Here's how the part is built. I have some questions about the finished solid (model axes, mm). A direction names the side the tool comes from. Round coordinates to 2 decimals unless told otherwise and drop trailing zeros. Write each loop counter-clockwise with the first axis right and the second up, starting at its lowest first coordinate (ties: lowest second). Pieces come first, ordered by that corner, then holes. Notation, with made-up numbers: (-37.75, -8.75) -> (17.25, -8.75) arc R14 ccw to (17.25, 7.25) -> close; hole circle Ø1 at (48, 10). An arc over 180 degrees is marked (long way). Put each result on its own line as item: value. Start each with the question number.
1. Suppose I cut it at D-D (x = 0). Please give me the cut outline in (y, z), then the cut area to 3 significant figures.
2. I need wall thicknesses on probe 1 along Y at (x, z) = (-7.25, -5.25); probe 2 along Y at (x, z) = (4.5, 4.5); probe 3 along X at (y, z) = (29, 0.25). Which ranges of each line are inside material? Lowest first, please. Write a range as from..to.
3. Suppose I cut it at B-B (z = 0). Please give me the cut outline in (x, y), then the cut area to 3 significant figures.
4. Which directions (+Z, -Z, +X, -X, +Y, -Y) give clear straight access to the entire face, cutting with the end or side of a thin tool? Please do faces 1 (the face through (0, 0, 0)), 2 (the face through (-6.324, 8.381, -4.032)), 3 (the face through (3, 47.5, 3)).
5. For pin 1 (4 mm diameter, centred on y = 62.5, z = 0, fed in from +X); pin 2 (4 mm diameter, centred on x = 6, y = 23.5, fed in from +Z); pin 3 (2 mm diameter, centred on y = 48, z = 2.5, fed in from +X), each with a flat end and sliding along its axis, tell me the tip position at first contact or that it passes through.
6. Suppose I cut it at C-C (y = 44.5). Please give me the cut outline in (x, z), then the cut area to 3 significant figures.
7. Suppose I cut it at A-A (x = -6). Please give me the cut outline in (y, z), then the cut area to 3 significant figures.
```python
from build123d import *


with BuildPart() as part:
    # Szkic1 → Obrót1 (revolve)
    with BuildSketch(Plane.XY, mode=Mode.PRIVATE) as obr_t1_sk:
        Polygon((4, 47.5), (7.5, 47.5), (7.5, 30.5), (10, 30.5), (10, 17), (7.5, 17), (7.5, 0), (0, 0), (0, 47.5), (0, 82.5), (4, 82.5), align=None)
    revolve(obr_t1_sk.sketch.rotate(Axis((0, 0, 0), (0, 1, 0)), 90), axis=Axis((0, 0, 0), (0, 1, 0)))


solid = part.part
```
Verdict:
1. outline: (0, -7.5) -> (17, -7.5) -> (17, -10) -> (30.5, -10) -> (30.5, -7.5) -> (47.5, -7.5) -> (47.5, -4) -> (82.5, -4) -> (82.5, 4) -> (47.5, 4) -> (47.5, 7.5) -> (30.5, 7.5) -> (30.5, 10) -> (17, 10) -> (17, 7.5) -> (0, 7.5) -> close
1. area: 1,060 mm^2
2. probe 1: y = 17..30.5
2. probe 2: y = 0..47.5
2. probe 3: x = -10..10
3. outline: (-10, 17) -> (-7.5, 17) -> (-7.5, 0) -> (7.5, 0) -> (7.5, 17) -> (10, 17) -> (10, 30.5) -> (7.5, 30.5) -> (7.5, 47.5) -> (4, 47.5) -> (4, 82.5) -> (-4, 82.5) -> (-4, 47.5) -> (-7.5, 47.5) -> (-7.5, 30.5) -> (-10, 30.5) -> close
3. area: 1,060 mm^2
4. face 1: +Z, -Z, +X, -X, -Y
4. face 2: -Y
4. face 3: +Y
5. pin 1: stops at x = 4
5. pin 2: stops at z = 9.17
5. pin 3: stops at x = 7.32
6. outline: circle Ø15 at (0, 0)
6. area: 177 mm^2
7. outline: (0, -4.5) -> (17, -4.5) -> (17, -8) -> (30.5, -8) -> (30.5, -4.5) -> (47.5, -4.5) -> (47.5, 4.5) -> (30.5, 4.5) -> (30.5, 8) -> (17, 8) -> (17, 4.5) -> (0, 4.5) -> close
7. area: 522 mm^2
